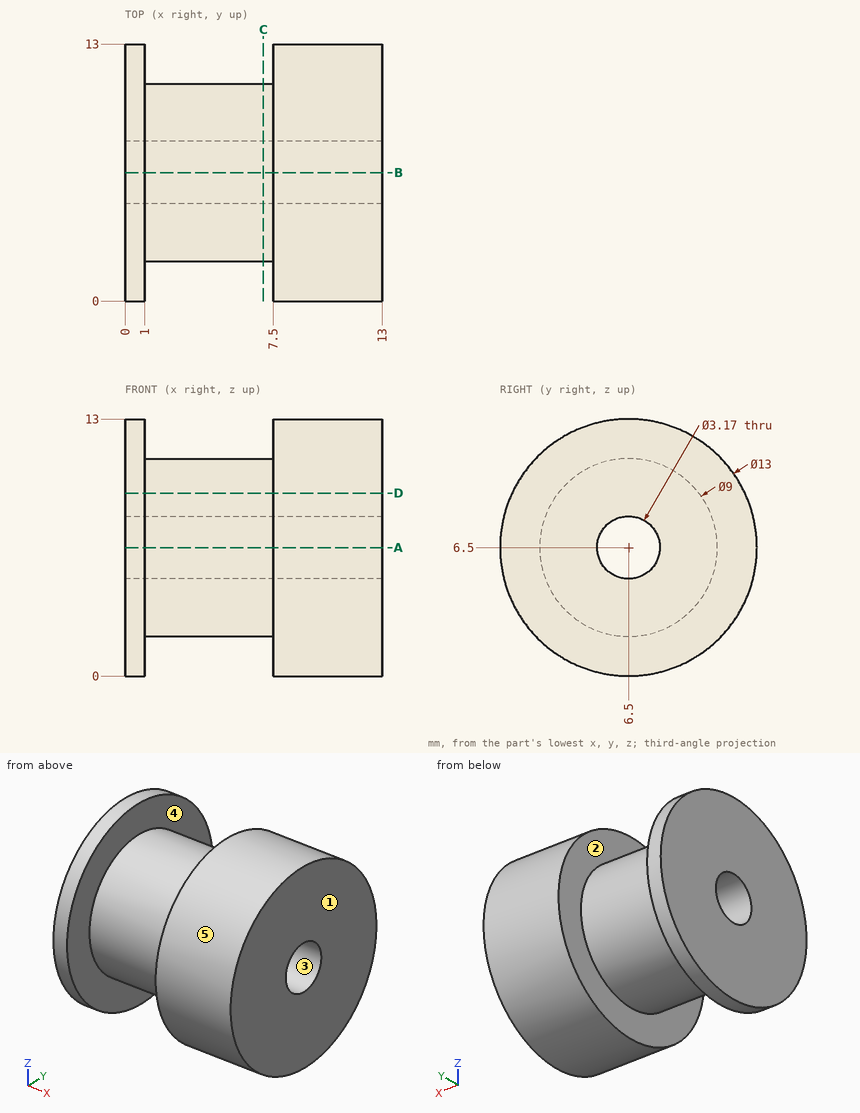
Here's the drawing with two shaded views (mm, measured from the low corner). I have some questions. A direction names the side the tool comes from. Round coordinates to 2 decimals unless told otherwise and drop trailing zeros. Loops run counter-clockwise (first coordinate to the right, second up) from the corner with the lowest first, then second, coordinate; pieces in that order, holes last.
Item 1: Will these pins go through, and if not, where does the flat tip stop? pin 1 Ø1 at (x, z) = (9.5, 3) entering from -Y; pin 2 Ø2 at (x, y) = (5, 11) entering from -Z; pin 3 Ø2 at (x, y) = (7, 4.5) entering from +Z.
Item 2: If we mould it in two halves opening along Z, with no side actions, what happens to the marked faces 3, 4 and 5? For each: +Z half, -Z half, draft (parallel to the pull), parting line (faces both ways), or undercut.
Item 3: Which directions (+Z, -Z, +X, -X, +Y, -Y) give clear straight access to the entire face, cutting with the end or side of a thin tool? Please do the marked faces 1 and 2.
Item 4: Suppose I cut it at A-A, the plane z = 6.5. Write out the boundary of the cut face in (x, y) (3 decimals).
Item 5: Please list where these lines run through material, in increasing order: L1, parallel to X at y = 4, z = 2.25; L2, parallel to Y at x = 2, z = 7; L3, parallel to Y at x = 4.25, z = 10.
Item 6: Suppose I cut it at D-D, the plane z = 9.25. Write out the boundary of the cut face in (x, y), then the cut area to 3 significant figures.
Item 7: Suppose I cut it at C-C, the plane x = 7. Write out the boundary of the cut face in (y, z) (3 decimals), then the cut area to 3 significant figures.
Reported:
1. pin 1: stops at y = 0.73
1. pin 2: stops at z = 3.67
1. pin 3: stops at z = 12.9
2. face 3: undercut
2. face 4: draft
2. face 5: parting line
3. face 1: +Z, -Z, +X, +Y, -Y
3. face 2: none
4. outline: (0, 0) - (1, 0) - (1, 2) - (7.5, 2) - (7.5, 0) - (13, 0) - (13, 4.915) - (0, 4.915) - close; (0, 8.085) - (13, 8.085) - (13, 13) - (7.5, 13) - (7.5, 11) - (1, 11) - (1, 13) - (0, 13) - close
5. L1: x = 0 to 1, 7.5 to 13
5. L2: y = 2.03 to 5, 8 to 10.97
5. L3: y = 3.67 to 9.33
6. outline: (0, 0.61) - (1, 0.61) - (1, 2.94) - (7.5, 2.94) - (7.5, 0.61) - (13, 0.61) - (13, 12.39) - (7.5, 12.39) - (7.5, 10.06) - (1, 10.06) - (1, 12.39) - (0, 12.39) - close
6. area: 123 mm2
7. outline: circle Ø9 at (6.5, 6.5); hole circle Ø3.17 at (6.5, 6.5)
7. area: 55.7 mm2
